The listing builds one solid part. Answer for the finished solid, in the listing's coordinates (mm). A direction names the side the tool comes from. Give positions to 0.01 mm unless a question says otherwise; leave off trailing zeros. Write each loop counter-clockwise with the first axis right and the second up, starting at its lowest first coordinate (ties: lowest second). Pieces come first, ordered by that corner, then holes. Notation, with made-up numbers: M 68,41.5 L 87,41.5 A32 ccw 87,80.5 Z; hole C 57,61 d1. An arc over 180 degrees is marked long. Answer as a JSON object with one key per item and string values.
```python
from build123d import *

# Parameters (mm, degrees)
SKETCH1_W           = 64.05
SKETCH1_H           = 52.6
BOSS_EXTRUDE1_DEPTH = 1.6
SKETCH2_W           = 64.05
SKETCH2_H           = 52.6
SKETCH2_W_2         = 60.05
SKETCH2_H_2         = 48.6
BOSS_EXTRUDE2_DEPTH = 3
SKETCH6_W           = 62.05
SKETCH6_H           = 50.6
SKETCH6_W_2         = 60.05
SKETCH6_H_2         = 48.6
BOSS_EXTRUDE6_DEPTH = 2
CUT_EXTRUDE2_DEPTH  = 2
FILLET2_R           = 0.2
SKETCH11_R          = 2
BOSS_EXTRUDE7_DEPTH = 3
SKETCH12_R          = 0.75
CUT_EXTRUDE3_DEPTH  = 2
FILLET4_R           = 1
BOSS_EXTRUDE8_DEPTH = 3
FILLET5_R           = 1
CHAMFER2_SIZE       = 0.2


with BuildPart() as part:
    # Sketch1 → Boss-Extrude1 (new body)
    with BuildSketch(Plane.XY):
        with Locations((29.525, 23.8)):
            Rectangle(SKETCH1_W, SKETCH1_H)
    extrude(amount=BOSS_EXTRUDE1_DEPTH)

    # Sketch2 → Boss-Extrude2 (add)
    with BuildSketch(Plane.XY.offset(1.6)):
        with Locations((29.525, 23.8)):
            Rectangle(SKETCH2_W, SKETCH2_H)
        with Locations((29.525, 23.8)):
            Rectangle(SKETCH2_W_2, SKETCH2_H_2, mode=Mode.SUBTRACT)
    extrude(amount=BOSS_EXTRUDE2_DEPTH)

    # Sketch6 → Boss-Extrude6 (add)
    with BuildSketch(Plane.XY.offset(4.6)):
        with Locations((29.525, 23.8)):
            Rectangle(SKETCH6_W, SKETCH6_H)
        with Locations((29.525, 23.8)):
            Rectangle(SKETCH6_W_2, SKETCH6_H_2, mode=Mode.SUBTRACT)
    extrude(amount=BOSS_EXTRUDE6_DEPTH)

    # Sketch9 → Cut-Extrude2 (cut)
    with BuildSketch(Plane(origin=(0, 0, 0), x_dir=(-1, 0, 0), z_dir=(0, 0, -1))):
        Polygon((-40.55, 27.6), (-54.55, 27.6), (-54.55, 25.1), (-57.55, 25.1), (-57.55, 33.1), (-54.55, 33.1), (-54.55, 30.6), (-40.55, 30.6), (-40.55, 31.6), (-53.55, 31.6), (-53.55, 34.1), (-58.55, 34.1), (-58.55, 24.1), (-53.55, 24.1), (-53.55, 26.6), (-40.55, 26.6), align=None)
    extrude(amount=-CUT_EXTRUDE2_DEPTH, mode=Mode.SUBTRACT)

    # Fillet2
    fillet2_edges = [part.edges().sort_by_distance(p)[0] for p in [
        (40.55, 27.6, 0.8),
        (40.55, 26.6, 0.8),
        (53.55, 26.6, 0.8),
        (53.55, 24.1, 0.8),
        (58.55, 24.1, 0.8),
        (58.55, 34.1, 0.8),
        (53.55, 34.1, 0.8),
        (53.55, 31.6, 0.8),
        (40.55, 31.6, 0.8),
        (40.55, 30.6, 0.8),
        (54.55, 30.6, 0.8),
        (54.55, 33.1, 0.8),
        (57.55, 33.1, 0.8),
        (57.55, 25.1, 0.8),
        (54.55, 25.1, 0.8),
        (54.55, 27.6, 0.8),
    ]]
    fillet(fillet2_edges, radius=FILLET2_R)

    # Sketch11 → Boss-Extrude7 (add)
    with BuildSketch(Plane.XY.offset(1.6)):
        with Locations(Location((1.6, 1.6, 0), (0, 0, 180))):
            Circle(SKETCH11_R)
        with Locations(Location((57.45, 1.6, 0), (0, 0, 180))):
            Circle(SKETCH11_R)
        with Locations(Location((44.05, 39.6, 0), (0, 0, 180))):
            Circle(SKETCH11_R)
        with Locations(Location((2.5, 39.6, 0), (0, 0, 180))):
            Circle(SKETCH11_R)
    extrude(amount=BOSS_EXTRUDE7_DEPTH)

    # Sketch12 → Cut-Extrude3 (cut)
    with BuildSketch(Plane.XY.offset(4.6)):
        with Locations((2.5, 39.6)):
            Circle(SKETCH12_R)
        with Locations((1.6, 1.6)):
            Circle(SKETCH12_R)
        with Locations((57.45, 1.6)):
            Circle(SKETCH12_R)
        with Locations((44.05, 39.6)):
            Circle(SKETCH12_R)
    extrude(amount=-CUT_EXTRUDE3_DEPTH, mode=Mode.SUBTRACT)

    # Fillet4
    fillet4_edges = [part.edges().sort_by_distance(p)[0] for p in [
        (59.55, 48.1, 4.1),
        (-0.5, 48.1, 4.1),
        (-1.5, -1.5, 5.6),
        (60.55, -1.5, 5.6),
        (60.55, 49.1, 5.6),
        (-1.5, 49.1, 5.6),
        (-2.5, 50.1, 2.3),
        (61.55, 50.1, 2.3),
        (61.55, -2.5, 2.3),
        (-2.5, -2.5, 2.3),
    ]]
    fillet(fillet4_edges, radius=FILLET4_R)

    # Sketch13 → Boss-Extrude8 (add)
    with BuildSketch(Plane.XY.offset(1.6)):
        with BuildLine():
            Line((1.6, 3.6), (-0.5, 3.6))
            Line((-0.5, 3.6), (-0.5, -0.5))
            Line((-0.5, -0.5), (3.6, -0.5))
            Line((3.6, -0.5), (3.6, 1.6))
            ThreePointArc((3.6, 1.6), (0.185786438, 0.185786438), (1.6, 3.6))
        make_face()
    boss_extrude8 = extrude(amount=BOSS_EXTRUDE8_DEPTH)

    # Mirror1: Boss-Extrude8 across plane
    add(boss_extrude8.mirror(Plane(origin=(29.525, 0, 0), x_dir=(0, 0, 1), z_dir=(1, 0, 0))))

    # Fillet5
    fillet5_edges = [part.edges().sort_by_distance(p)[0] for p in [
        (-0.5, -0.5, 5.6),
        (59.55, -0.5, 5.6),
        (-0.5, 3.6, 3.1),
        (3.6, -0.5, 3.1),
        (59.55, 3.6, 3.1),
        (55.45, -0.5, 3.1),
    ]]
    fillet(fillet5_edges, radius=FILLET5_R)

    # Chamfer2
    chamfer2_edges = [part.edges().sort_by_distance(p)[0] for p in [
        (1.75, 39.6, 4.6),
        (0.85, 1.6, 4.6),
        (56.7, 1.6, 4.6),
        (43.3, 39.6, 4.6),
    ]]
    chamfer(chamfer2_edges, length=CHAMFER2_SIZE)


solid = part.part
```
1. Consider line 1 along Y through (x, z) = (55, 0.75); line 2 along X through (y, z) = (39.6, 3.1); line 3 along Y through (x, z) = (44, 0.5). Determine where each line is inside the solid, lowest interval first.
Verdict:
{"line 1": "y = -2.5 to 24.1, 25.1 to 33.1, 34.1 to 50.1", "line 2": "x = -2.5 to -0.5, 0.5 to 1.75, 3.25 to 4.5, 42.05 to 43.3, 44.8 to 46.05, 59.55 to 61.55", "line 3": "y = -2.5 to 26.6, 27.6 to 30.6, 31.6 to 50.1"}
2. The mould has two halves that part along Y. Classify faces 1 (the flat face through (29.4, 48.3, 6.6)), 2 (the flat face through (47, 31.6, 1)): released by +Y, released by -Y, zero draft, split by the parting line, or undercut.
Verdict:
{"face 1": "zero draft", "face 2": "undercut"}
3. A cutting plane is placed at D-D, the plane x = 32. Give the vertices of the cut face in (y, z).
Verdict:
{"outline": "M -2.5,0 L 50.1,0 L 50.1,4.6 L 49.1,4.6 L 49.1,6.6 L 48.1,6.6 L 48.1,1.6 L -0.5,1.6 L -0.5,6.6 L -1.5,6.6 L -1.5,4.6 L -2.5,4.6 Z"}
4. For faces 3 (the cylindrical face through (44.74, 39.31, 3.51)), 4 (the flat face through (57.55, 29, 1)), determine the directions among +Z, -Z, +X, -X, +Y, -Y from which every point of the face is accessible in a straight line to the end or side of a thin tool.
Verdict:
{"face 3": "+Z", "face 4": "+Z, -Z"}
5. A cutting plane is placed at C-C, the plane y = 12. Give the vertices of the cut face in (x, z).
Verdict:
{"outline": "M -2.5,0 L 61.55,0 L 61.55,4.6 L 60.55,4.6 L 60.55,6.6 L 59.55,6.6 L 59.55,1.6 L -0.5,1.6 L -0.5,6.6 L -1.5,6.6 L -1.5,4.6 L -2.5,4.6 Z"}
6. A cutting plane is placed at A-A, the plane z = 3.5. Count the separate pieces of the cut face and the enclosed holes in it, plus the area to 3 significant figures.
Verdict:
{"separate pieces": "3", "enclosed holes": "5", "area": "501 mm2"}
7. Flat-ended cylindrical pins translate along their axes: pin 1 (2.5 mm diameter, centred on x = 1.5, y = 1.5, fed in from +Z); pin 2 (2 mm diameter, centred on x = 44.05, y = 39.6, fed in from -Z); pin 3 (4 mm diameter, centred on x = 45.5, y = 18, fed in from +Z); pin 4 (1 mm diameter, centred on x = 30, z = 5.5, fed in from +Y). Find the tip coordinate at first contact, or state that the pin passes through.
Verdict:
{"pin 1": "stops at z = 4.6", "pin 2": "stops at z = 0", "pin 3": "stops at z = 1.6", "pin 4": "stops at y = 49.1"}
